Autodesk Inventor part; units mm, degrees
ref_plane "bnt_s_1_XY" through (0, 0, 0) normal (-1, 0, 0) x (0, 0, -1)
ref_plane "bnt_s_1_YZ" through (0, 0, 0) normal (0, 0, -1) x (0, -1, 0)
ref_plane "bnt_s_1_ZX" through (0, 0, 0) normal (0, -1, 0) x (-1, 0, 0)
sketch "Sketch_1" plane through (0, 0, 0) normal (0, 0, 1) x (1, 0, 0)
  line L0 (1263, 0) -> (5, 0)
  line L1 (5, 0) -> (5, 10)
  line L2 (5, 10) -> (1263, 10)
  line L3 (1263, 10) -> (1263, 0)
  line L4 (1263, 0) -> (5, 0)
revolve "Revolution1" add sketch "Sketch_1" angle 360 about axis through (1263, 0, 0) along (1, 0, 0)
thread "Thread1"
sketch "Sketch_2" plane through (0, 0, 0) normal (0, 1, 0) x (-1, 0, 0)
  line L0 (-5, 0) -> (0, 0)
  line L1 (0, 0) -> (0, -9)
  line L2 (0, -9) -> (-1, -10)
  line L3 (-1, -10) -> (-4.8, -10)
  line L4 (-4.8, -10) -> (-4.8, -8)
  line L5 (-4.8, -8) -> (-5, -8)
  line L6 (-5, -8) -> (-5, 0)
  line L7 (-5, 0) -> (0, 0)
revolve "Revolution2" add sketch "Sketch_2" angle 360 about axis through (5, 0, 0) along (1, 0, 0)
sketch "Sketch_3" plane through (0, 0, 0) normal (0, 1, 0) x (-1, 0, 0)
  line L0 (-1268, 0) -> (-1263, 0)
  line L1 (-1263, 0) -> (-1263, -8)
  line L2 (-1263, -8) -> (-1263.2, -8)
  line L3 (-1263.2, -8) -> (-1263.2, -10)
  line L4 (-1263.2, -10) -> (-1267, -10)
  line L5 (-1267, -10) -> (-1268, -9)
  line L6 (-1268, -9) -> (-1268, 0)
  line L7 (-1268, 0) -> (-1263, 0)
revolve "Revolution3" add sketch "Sketch_3" angle 360 about axis through (1268, 0, 0) along (1, 0, 0)
ref_plane "bnt_s_1_XY" through (0, 0, 0) normal (-1, 0, 0) x (0, 0, -1)
ref_plane "bnt_s_1_YZ" through (0, 0, 0) normal (0, 0, -1) x (0, -1, 0)
ref_plane "bnt_s_1_ZX" through (0, 0, 0) normal (0, -1, 0) x (-1, 0, 0)
properties part number "BNT 2010-2.61200 Shaft"
Design review of the part built by this model. Coordinates are the model's own, in mm. A direction names the side the tool comes from. Coordinates: 2 decimals unless noted, no trailing zeros. Loops run counter-clockwise (first coordinate to the right, second up) from the corner with the lowest first, then second, coordinate; pieces in that order, holes last. Notation, with made-up numbers: (-28, -0.75) - (-20, -0.75) arc R22 ccw to (-20, 22.25) - close; hole circle Ø3 at (80.5, 47.25). An arc over 180 degrees is marked (long way). Use CSV: the item, a comma, the result in double quotes. Start each with the question number.
1) For pin 1 Ø10 at (x, z) = (288.5, 7.5) entering from -Y; pin 2 Ø3 at (y, z) = (-7, 8) entering from -X; pin 3 Ø6 at (x, y) = (512, 7) entering from +Z, all flat-tipped, find the tip position at first contact; note any pin that passes through.
2) Consider section A-A on x = 927.5. Write out the cut boundary in (y, z).
3) Wall thickness on L1, parallel to X at y = 3.75, z = -7.75; L2, parallel to X at y = -7, z = 6.75; L3, parallel to Y at x = 206.5, z = -0.75: over which ranges is each line inside the solid? List them lowest first. Write a range as from..to.
4) Tool access review of faces 1 (the cylindrical face through (642.81, -2.17, -9.76)), 2 (the flat face through (5, 0, 8.2)): name each direction out of +Z, -Z, +X, -X, +Y, -Y from which nothing blocks a thin tool from reaching the whole face with its end or side.
5) The part is to be moulded in two halves that separate along X. For faces 3 (the flat face through (4.8, 8.2, 0)), 4 (the cylindrical face through (2.93, -9.76, 2.17)), say which applies: +X half, -X half, draft (parallel to the pull), parting line (faces both ways), or undercut.
Geometry says:
1,pin 1,"y = -9.68"
1,pin 2,"x = 0.13"
1,pin 3,"z = 9.17"
2,outline,"circle Ø20 at (0, 0)"
3,L1,"0..4.8, 5..1263, 1263.2..1268"
3,L2,"0.72..4.8, 5..1263, 1263.2..1267.28"
3,L3,"-9.97..9.97"
4,face 1,"+X, -X"
4,face 2,"none"
5,face 3,"undercut"
5,face 4,"draft"
